Input: part model. Units: mm. Frame: model coordinates. A direction names the side the tool comes from. Give positions to 0.01 mm unless a question says otherwise; leave off trailing zeros. Loops run counter-clockwise (first coordinate to the right, second up) from the corner with the lowest first, then second, coordinate; pieces in that order, holes last. Notation, with made-up numbers: (76.5, -25.5) - (113.5, -25.5) arc R27 ccw to (113.5, 12.5) - close; hole circle Ø7 at (40, -4.5). An arc over 180 degrees is marked (long way). One line per item, written item: value.
from build123d import *

# Parameters (mm, degrees)
SKETCH3_W           = 19.05
SKETCH3_H           = 25.4
BOSS_EXTRUDE1_DEPTH = 20.32
SKETCH4_W           = 13.97
SKETCH4_H           = 20.32
CUT_EXTRUDE1_DEPTH  = 17.78
CUT_EXTRUDE3_START  = -2.54
CUT_EXTRUDE3_DEPTH  = 13.97


with BuildPart() as part:
    # Sketch3 → Boss-Extrude1 (new body)
    with BuildSketch(Plane(origin=(0, 0, 0), x_dir=(1, 0, 0), z_dir=(0, 1, 0))):
        with Locations((9.525, 12.7)):
            Rectangle(SKETCH3_W, SKETCH3_H)
    extrude(amount=BOSS_EXTRUDE1_DEPTH)

    # Sketch4 → Cut-Extrude1 (cut)
    with BuildSketch(Plane(origin=(0, 20.32, 0), x_dir=(1, 0, 0), z_dir=(0, 1, 0))):
        with Locations((9.525, 12.7)):
            Rectangle(SKETCH4_W, SKETCH4_H)
    extrude(amount=-CUT_EXTRUDE1_DEPTH, mode=Mode.SUBTRACT)

    # Sketch6 → Cut-Extrude3 (cut)
    with BuildSketch(Plane.ZY.offset(CUT_EXTRUDE3_START)):
        Polygon((-2.562657446, 20.32), (-0.635, 20.32), (-2.562657446, 12.678976029), align=None)
    extrude(amount=-CUT_EXTRUDE3_DEPTH, mode=Mode.SUBTRACT)


solid = part.part
Item 1: Access query for faces 1 (the face through (9, 8, -2.54)), 2 (the face through (9, 10, -25.4)). Directions: +Z, -Z, +X, -X, +Y, -Y. A direction counts if a zero-diameter tool reaches every point of the face in a straight line with its end or side. Return the directions, or none.
Verdict:
face 1: +Y
face 2: -Z, +X, -X, +Y, -Y
Item 2: Section B-B, the plane z = -22.5. Output: boundary loops of the cut face in (x, y), and give its area (3 significant figures).
Verdict:
outline: (0, 0) - (19.05, 0) - (19.05, 20.32) - (16.51, 20.32) - (16.51, 2.54) - (2.54, 2.54) - (2.54, 20.32) - (0, 20.32) - close
area: 139 mm^2
Item 3: Draft query along X for faces 3 (the face through (17, 20.32, -15)), 4 (the face through (16.51, 12, -12)), 5 (the face through (2.54, 12, -12)), 6 (the face through (19.05, 10, -13)). Return one class per face: pulls with the +X half, pulls with the -X half, needs draft (parallel to the pull), parting line crosses it, or undercut.
Verdict:
face 3: needs draft
face 4: undercut
face 5: undercut
face 6: pulls with the +X half
Item 4: Section C-C, the plane x = 3. Output: boundary loops of the cut face in (y, z) (3 decimals).
Verdict:
outline: (0, -25.4) - (20.32, -25.4) - (20.32, -22.86) - (2.54, -22.86) - (2.54, -2.54) - (12.769, -2.54) - (20.32, -0.635) - (20.32, 0) - (0, 0) - close
Item 5: Material intervals for L1, parallel to X at y = 19.75, z = -22; L2, parallel to Z at x = 13.25, y = 10.75; L3, parallel to Z at x = 14.25, y = 13.75, sorted ascending.
Verdict:
L1: x = 0 to 2.54, 16.51 to 19.05
L2: z = -25.4 to -22.86, -2.54 to 0
L3: z = -25.4 to -22.86, -2.29 to 0
Item 6: Section A-A, the plane y = 7.5. Output: boundary loops of the cut face in (x, z), and give its area (3 significant figures).
Verdict:
outline: (0, -25.4) - (19.05, -25.4) - (19.05, 0) - (0, 0) - close; hole (2.54, -22.86) - (16.51, -22.86) - (16.51, -2.54) - (2.54, -2.54) - close
area: 200 mm^2
